Input: part model. Units: mm. Frame: model coordinates. A direction names the side the tool comes from. Coordinates: 2 decimals unless noted, no trailing zeros. Loops run counter-clockwise (first coordinate to the right, second up) from the corner with the lowest first, then second, coordinate; pieces in that order, holes last. Notation, with made-up numbers: (78.5, 85) -> (106.5, 85) arc R17 ccw to (106.5, 113) -> close; hole circle Ø5 at (30, 59.25). An arc over 180 degrees is marked (long way). Put each result on its own line as item: value. Start each with the question number.
1) Pull-direction query (X, two-part tool) for faces 6 (the flat face through (0, -6, 3.175)), 7 (the cylindrical face through (71.86, -72.93, 1.57)), 8 (the flat face through (-54, -39, 2)); classes: pulls with the +X half, pulls with the -X half, needs draft (parallel to the pull), parting line crosses it, or undercut.
2) Contact query for flat-ended pins moving along their axis: P1, Ø1.6, axis at x = 63, z = 1, coming from the -Y side; P2, Ø1, axis at x = 62, z = 1.5, coming from the +Y side; P3, Ø1.6, axis at x = 79, z = 1, coming from the -Y side; P4, Ø1.8, axis at x = 18, y = -22.5, coming from the -Z side. Output: stop coordinate, or through.
3) Material intervals for L1, parallel to Y at x = -6.5, z = 1.9; L2, parallel to Y at x = 75, z = 2.2; L3, parallel to Y at x = -62, z = 2.8, sorted ascending.
4) Cut plane C-C (z = 0.55). State how many separate pieces and enclosed holes the cut face has, plus the area to 3 significant figures.
5) Set-up query: faces 1 (the flat face through (31.12, 48.18, 1.57)), 2 (the cylindrical face through (80.962, -81.661, 1.565)), 3 (the flat face through (-54, 39, 2)), 4 (the flat face through (30.419, -47.535, 1.565)), 5 (the flat face through (46.521, 33.545, 1.565)). Return all of +Z, -Z, +X, -X, +Y, -Y with unobstructed straight access to the full face (end or side cutting, diameter ignored); none if empty.
6) Cut plane B-B (y = 52). Return the cut outline in (x, z) (3 decimals).
7) Cut plane A-A (x = -45). Return the cut outline in (y, z) (3 decimals), plus the area to 4 significant figures.
8) Cut plane D-D (y = 7.5). Return the cut outline in (x, z) (3 decimals).
from build123d import *

# Parameters (mm, degrees)
F0_R     = 2.5
F0_R_2   = 1.5
F0_W     = 25
F0_H     = 3
F1_DEPTH = 3.175


# Not quite as in the source:
# - ends of sketch curves that miss each other by under 0.0002 mm in the source are joined


with BuildPart() as f1:
    # F0 (on Top) → F1 (new body)
    with BuildSketch(Plane.XY):
        with BuildLine():
            Line((-10.0000000587, 25), (-55.7106781187, 70.7106779065))
            ThreePointArc((-55.7106781187, 70.7106779065), (-81.3172799026, 81.3172797703), (-70.7106779065, 55.7106781187))
            Line((-70.7106779065, 55.7106781187), (-37, 22.0000003253))
            Line((-37, 22.0000003253), (-37, -22.0000003253))
            Line((-37, -22.0000003253), (-70.7106779065, -55.7106781187))
            ThreePointArc((-70.7106779065, -55.7106781187), (-81.3172798365, -81.3172798365), (-55.7106781187, -70.7106779065))
            Line((-55.7106781187, -70.7106779065), (-10.0000000587, -25))
            Line((-10.0000000587, -25), (5.8262266936, -25))
            Line((5.8262266936, -25), (55.7106781187, -70.7106780935))
            ThreePointArc((55.7106781187, -70.7106780935), (81.3172798365, -81.3172798365), (70.7106780935, -55.7106781187))
            Line((70.7106780935, -55.7106781187), (23, -11.9918965954))
            Line((23, -11.9918965954), (23, 11.9918965954))
            Line((23, 11.9918965954), (70.7106780935, 55.7106781187))
            ThreePointArc((70.7106780935, 55.7106781187), (81.3172798365, 81.3172798365), (55.7106781187, 70.7106779065))
            Line((55.7106781187, 70.7106779065), (5.8262266936, 25))
            Line((5.8262266936, 25), (-10.0000000587, 25))
        make_face()
        with BuildLine():
            Line((-72.210678, -81.1510407925), (-72.210678, -76.1510407925))
            ThreePointArc((-72.210678, -76.1510407925), (-70.710678, -74.6510407925), (-69.210678, -76.1510407925))
            Line((-69.210678, -76.1510407925), (-69.210678, -81.1510407925))
            ThreePointArc((-69.210678, -81.1510407925), (-70.710678, -82.6510407925), (-72.210678, -81.1510407925))
        make_face(mode=Mode.SUBTRACT)
        with BuildLine():
            Line((-81.1510407874, -69.2106756767), (-76.1510407874, -69.2106756935))
            ThreePointArc((-76.1510407874, -69.2106756935), (-74.6510407925, -70.7106782241), (-76.1510407975, -72.2106782191))
            Line((-76.1510407975, -72.2106782191), (-81.1510407975, -72.2106755673))
            ThreePointArc((-81.1510407975, -72.2106755673), (-82.6510407925, -70.7106781972), (-81.1510407874, -69.2106756767))
        make_face(mode=Mode.SUBTRACT)
        with Locations((-70.7106781187, -70.7106781187)):
            Circle(F0_R, mode=Mode.SUBTRACT)
        with BuildLine():
            Line((-60.2703154499, -72.210678035), (-65.2703154499, -72.2106780183))
            ThreePointArc((-65.2703154499, -72.2106780183), (-66.7703154448, -70.7106780132), (-65.2703154398, -69.2106780183))
            Line((-65.2703154398, -69.2106780183), (-60.2703154398, -69.210678035))
            ThreePointArc((-60.2703154398, -69.210678035), (-58.7703154448, -70.7106780401), (-60.2703154499, -72.210678035))
        make_face(mode=Mode.SUBTRACT)
        with BuildLine():
            Line((-69.210678035, -60.2703154398), (-69.2106780183, -65.2703154398))
            ThreePointArc((-69.2106780183, -65.2703154398), (-70.7106780132, -66.7703154448), (-72.2106780183, -65.2703154499))
            Line((-72.2106780183, -65.2703154499), (-72.210678035, -60.2703154499))
            ThreePointArc((-72.210678035, -60.2703154499), (-70.7106780401, -58.7703154448), (-69.210678035, -60.2703154398))
        make_face(mode=Mode.SUBTRACT)
        with Locations((-32.5, -13)):
            Circle(F0_R_2, mode=Mode.SUBTRACT)
        with Locations((-15.25, -15.25)):
            Circle(F0_R_2, mode=Mode.SUBTRACT)
        with BuildLine():
            Line((60.2703154398, -69.210678035), (65.2703154398, -69.2106780183))
            ThreePointArc((65.2703154398, -69.2106780183), (66.7703154448, -70.7106780132), (65.2703154499, -72.2106780183))
            Line((65.2703154499, -72.2106780183), (60.2703154499, -72.210678035))
            ThreePointArc((60.2703154499, -72.210678035), (58.7703154448, -70.7106780401), (60.2703154398, -69.210678035))
        make_face(mode=Mode.SUBTRACT)
        with BuildLine():
            ThreePointArc((69.210678, -76.1510407925), (70.710678, -74.6510407925), (72.210678, -76.1510407925))
            Line((72.210678, -76.1510407925), (72.210678, -81.1510407925))
            ThreePointArc((72.210678, -81.1510407925), (70.710678, -82.6510407925), (69.210678, -81.1510407925))
            Line((69.210678, -81.1510407925), (69.210678, -76.1510407925))
        make_face(mode=Mode.SUBTRACT)
        with Locations((70.7106781187, -70.7106781187)):
            Circle(F0_R, mode=Mode.SUBTRACT)
        with BuildLine():
            ThreePointArc((76.1510407975, -72.2106782191), (74.6510407925, -70.7106782241), (76.1510407874, -69.2106782191))
            Line((76.1510407874, -69.2106782191), (81.1510407874, -69.2106756767))
            ThreePointArc((81.1510407874, -69.2106756767), (82.6510407925, -70.7106781972), (81.1510407975, -72.2106782023))
            Line((81.1510407975, -72.2106782023), (76.1510407975, -72.2106782191))
        make_face(mode=Mode.SUBTRACT)
        with BuildLine():
            ThreePointArc((72.2106780183, -65.2703154499), (70.7106780132, -66.7703154448), (69.2106780183, -65.2703154398))
            Line((69.2106780183, -65.2703154398), (69.210678035, -60.2703154398))
            ThreePointArc((69.210678035, -60.2703154398), (70.7106780401, -58.7703154448), (72.210678035, -60.2703154499))
            Line((72.210678035, -60.2703154499), (72.2106780183, -65.2703154499))
        make_face(mode=Mode.SUBTRACT)
        with Locations((18, -22.5)):
            Circle(F0_R_2, mode=Mode.SUBTRACT)
        with Locations((0, -20.5)):
            Rectangle(F0_W, F0_H, mode=Mode.SUBTRACT)
        with Locations((15.25, -15.25)):
            Circle(F0_R_2, mode=Mode.SUBTRACT)
        with Locations((-32.5, 13)):
            Circle(F0_R_2, mode=Mode.SUBTRACT)
        with Locations((-15.25, 15.25)):
            Circle(F0_R_2, mode=Mode.SUBTRACT)
        with BuildLine():
            ThreePointArc((-72.2106780183, 65.2703154499), (-70.7106780132, 66.7703154448), (-69.2106780183, 65.2703154398))
            Line((-69.2106780183, 65.2703154398), (-69.210678035, 60.2703154398))
            ThreePointArc((-69.210678035, 60.2703154398), (-70.7106780401, 58.7703154448), (-72.210678035, 60.2703154499))
            Line((-72.210678035, 60.2703154499), (-72.2106780183, 65.2703154499))
        make_face(mode=Mode.SUBTRACT)
        with BuildLine():
            ThreePointArc((-76.1510407975, 72.2106782191), (-74.6510407925, 70.7106782241), (-76.1510407874, 69.2106782191))
            Line((-76.1510407874, 69.2106782191), (-81.1510407874, 69.2106782023))
            ThreePointArc((-81.1510407874, 69.2106782023), (-82.6510407925, 70.7106781972), (-81.1510407975, 72.2106782023))
            Line((-81.1510407975, 72.2106782023), (-76.1510407975, 72.2106782191))
        make_face(mode=Mode.SUBTRACT)
        with BuildLine():
            ThreePointArc((-68.9429111657, 72.4784450716), (-68.4009792874, 71.6673866996), (-68.2106781187, 70.7106781187))
            ThreePointArc((-68.2106781187, 70.7106781187), (-69.7539695377, 68.4009792874), (-72.4784450716, 68.9429111657))
            ThreePointArc((-72.4784450716, 68.9429111657), (-72.4784450716, 72.4784450716), (-68.9429111657, 72.4784450716))
        make_face(mode=Mode.SUBTRACT)
        with BuildLine():
            Line((-69.210678, 81.1510407925), (-69.210678, 76.1510407925))
            ThreePointArc((-69.210678, 76.1510407925), (-70.710678, 74.6510407925), (-72.210678, 76.1510407925))
            Line((-72.210678, 76.1510407925), (-72.210678, 81.1510407925))
            ThreePointArc((-72.210678, 81.1510407925), (-70.710678, 82.6510407925), (-69.210678, 81.1510407925))
        make_face(mode=Mode.SUBTRACT)
        with BuildLine():
            Line((-60.2703154398, 69.2106755095), (-65.2703154398, 69.2106754927))
            ThreePointArc((-65.2703154398, 69.2106754927), (-66.7703154448, 70.7106780132), (-65.2703154499, 72.2106780183))
            Line((-65.2703154499, 72.2106780183), (-60.2703154499, 72.2106754))
            ThreePointArc((-60.2703154499, 72.2106754), (-58.7703154448, 70.7106780401), (-60.2703154398, 69.2106755095))
        make_face(mode=Mode.SUBTRACT)
        with Locations((0, 20.5)):
            Rectangle(F0_W, F0_H, mode=Mode.SUBTRACT)
        with Locations((15.25, 15.25)):
            Circle(F0_R_2, mode=Mode.SUBTRACT)
        with Locations((18, 22.5)):
            Circle(F0_R_2, mode=Mode.SUBTRACT)
        with BuildLine():
            Line((69.210678035, 60.2703154398), (69.2106780183, 65.2703154398))
            ThreePointArc((69.2106780183, 65.2703154398), (70.7106780132, 66.7703154448), (72.2106780183, 65.2703154499))
            Line((72.2106780183, 65.2703154499), (72.210678035, 60.2703154499))
            ThreePointArc((72.210678035, 60.2703154499), (70.7106780401, 58.7703154448), (69.210678035, 60.2703154398))
        make_face(mode=Mode.SUBTRACT)
        with BuildLine():
            ThreePointArc((65.2703154499, 72.2106780183), (66.7703154448, 70.7106780132), (65.2703154398, 69.2106780183))
            Line((65.2703154398, 69.2106780183), (60.2703154398, 69.2106805606))
            ThreePointArc((60.2703154398, 69.2106805606), (58.7703154448, 70.7106780401), (60.2703154499, 72.210678035))
            Line((60.2703154499, 72.210678035), (65.2703154499, 72.2106780183))
        make_face(mode=Mode.SUBTRACT)
        with Locations((70.7106781187, 70.7106781187)):
            Circle(F0_R, mode=Mode.SUBTRACT)
        with BuildLine():
            Line((81.1510407874, 69.2106731512), (76.1510407874, 69.210673168))
            ThreePointArc((76.1510407874, 69.210673168), (74.6510407925, 70.7106782241), (76.1510407975, 72.2106782191))
            Line((76.1510407975, 72.2106782191), (81.1510407975, 72.2106729322))
            ThreePointArc((81.1510407975, 72.2106729322), (82.6510407925, 70.7106781972), (81.1510407874, 69.2106731512))
        make_face(mode=Mode.SUBTRACT)
        with BuildLine():
            Line((72.210678, 81.1510407925), (72.210678, 76.1510407925))
            ThreePointArc((72.210678, 76.1510407925), (70.710678, 74.6510407925), (69.210678, 76.1510407925))
            Line((69.210678, 76.1510407925), (69.210678, 81.1510407925))
            ThreePointArc((69.210678, 81.1510407925), (70.710678, 82.6510407925), (72.210678, 81.1510407925))
        make_face(mode=Mode.SUBTRACT)
    extrude(amount=F1_DEPTH)


solid = f1.part
Results found:
1. face 6: needs draft
1. face 7: undercut
1. face 8: pulls with the -X half
2. P1: stops at y = -84.02
2. P2: stops at y = 83.26
2. P3: stops at y = -83.71
2. P4: passes through
3. L1: y = -25 to -22, -19 to 19, 22 to 25
3. L2: y = -85.08 to -71.67, -69.75 to -56.34, 56.34 to 69.75, 71.67 to 85.08
3. L3: y = -82.92 to -72.21, -69.21 to -47, 47 to 69.21, 72.21 to 82.92
4. separate pieces: 1
4. enclosed holes: 30
4. area: 9,820 mm2
5. face 1: +Z, -Z, +Y
5. face 2: +Z, -Z
5. face 3: +Z, -Z, -X
5. face 4: +Z, -Z, -Y
5. face 5: +Z, -Z, +X
6. outline: (-67, 0) -> (-37, 0) -> (-37, 3.175) -> (-67, 3.175) -> close; (35.292, 0) -> (66.661, 0) -> (66.661, 3.175) -> (35.292, 3.175) -> close
7. outline: (-60, 0) -> (-30, 0) -> (-30, 3.175) -> (-60, 3.175) -> close; (30, 0) -> (60, 0) -> (60, 3.175) -> (30, 3.175) -> close
7. area: 190.5 mm2
8. outline: (-37, 0) -> (23, 0) -> (23, 3.175) -> (-37, 3.175) -> close
